Autodesk Inventor part; units mm, degrees
ref_plane "YZ Plane" through (0, 0, 0) normal (1, 0, 0) x (0, 1, 0)
ref_plane "XZ Plane" through (0, 0, 0) normal (0, 1, 0) x (-1, 0, 0)
ref_plane "XY Plane" through (0, 0, 0) normal (0, 0, 1) x (1, 0, 0)
sketch "Skizze1" plane through (0, 0, 0) normal (0, 0, 1) x (1, 0, 0)
  line L0 (0, 0) -> (0, 5.5)
  line L1 (0, 5.5) -> (5.6, 5.5)
  line L2 (5.6, 5.5) -> (5.6, 5)
  line L3 (5.6, 5) -> (13.6, 5)
  line L4 (13.6, 5) -> (13.6, 4.8)
  line L5 (13.6, 4.8) -> (14.7, 4.8)
  line L6 (14.7, 4.8) -> (14.7, 5)
  line L7 (14.7, 5) -> (15.3, 5)
  line L8 (15.8, 4.5) -> (15.8, 0)
  line L9 (15.8, 0) -> (0, 0)
  line L10 (0, 4) -> (-9.75, 4)
  line L11 (-11, 2.75) -> (-11, 0)
  line L12 (-11, 0) -> (0, 0)
  line L13 (15.3, 5) -> (15.8, 4.5)
  line L14 (-11, 2.75) -> (-9.75, 4)
  line L15 (1.5, 5.5) -> (1.5, 0) construction
  line L16 (13.6, 5) -> (13.6, 0) construction
  line L17 (4.6, 5.5) -> (4.6, 6)
  line L18 (4.6, 6) -> (0, 6)
  line L19 (0, 6) -> (0, 5.5)
  point P0 (15.8, 5)
  point P1 (-11, 4)
  dimension "d0" = 9.6
  dimension "d1" = 0.5
  dimension "d2" = 0.5
  dimension "d3" = 1.1
  dimension "d4" = 10
  dimension "d5" = 0.6
  dimension "d6" = 11
  dimension "d8" = 8
  dimension "d9" = 1.25
  dimension "d10" = 1.25
  dimension "d11" = 11
  dimension "d12" = 4.1
  dimension "d13" = 1.5
  dimension "d14" = 12.1
  dimension "d15" = 0
  dimension "d22" = 1
  dimension "d23" = 12
revolve "Umdrehung1" add sketch "Skizze1" angle 360 about axis through (15.8, 0, 0) along (-1, 0, 0) contours L12 L11 L14 L10 L0 | L0 L1 L2 L3 L4 L5 L6 L7 L13 L8 L9
thread "Gewinde1"
chamfer "Fase1" distance 0.1 angle 45 2 edges at (5.6, -5.5, 0) (0, -5.5, 0)
equation "\"d12\" = Bearing_StepThickness + SupportLink_Proximal_DistStep_Thickness"
equation "\"d14\" = Link_Thickness + SupportLink_Proximal_DistStep_Thickness"
equation "\"SupportLink_Proximal_DistStep_Thickness\" = 2.1"
properties part number "ParallelMech_SupportLink_Proximal_JointShaft"
Here's how the part is built. I have some questions about the finished solid (model axes, mm). A direction names the side the tool comes from. Round coordinates to 2 decimals unless told otherwise and drop trailing zeros. Order: outer loops, then holes, each group sorted by start corner. A loop starts at its lowest first (then second) coordinate and runs counter-clockwise, first axis right, second up. Notation, with made-up numbers: (-31.75, 7.5) -> (-17.75, 7.5) arc R26 cw to (-17.75, 24.5) -> close; hole circle Ø1 at (14, -35.75). An arc over 180 degrees is marked (long way). Use CSV: the item, a comma, the result in double quotes.
1. I need wall thicknesses on line 1 along Z through (x, y) = (-1.25, 0); line 2 along X through (y, z) = (2.5, -3.5); line 3 along X through (y, z) = (-4.75, 2.25). Which ranges of each line are inside material? Lowest first, please.
Recorded:
line 1,"z = -4 to 4"
line 2,"x = 0 to 15.8"
line 3,"x = 0 to 5.6"
2. I want a section at A-A on z = 0. List the corners of the cut face in (x, y) for me.
Recorded:
outline,"(-11, -2.75) -> (-9.75, -4) -> (0, -4) -> (0, -5.4) -> (0.1, -5.5) -> (5.5, -5.5) -> (5.6, -5.4) -> (5.6, -5) -> (13.6, -5) -> (13.6, -4.8) -> (14.7, -4.8) -> (14.7, -5) -> (15.3, -5) -> (15.8, -4.5) -> (15.8, 4.5) -> (15.3, 5) -> (14.7, 5) -> (14.7, 4.8) -> (13.6, 4.8) -> (13.6, 5) -> (5.6, 5) -> (5.6, 5.4) -> (5.5, 5.5) -> (0.1, 5.5) -> (0, 5.4) -> (0, 4) -> (-9.75, 4) -> (-11, 2.75) -> close"
3. I want a section at D-D on x = -0.75. List the corners of the cut face in (y, z) for me.
Recorded:
outline,"circle Ø8 at (0, 0)"
4. I want a section at C-C on x = 6.25. List the corners of the cut face in (y, z) for me.
Recorded:
outline,"circle Ø10 at (0, 0)"
5. I'm going to push flat-ended pins straight in: P1, Ø3, axis at x = -3.5, y = 1.5, coming from the -Z side; P2, Ø5, axis at x = -3, z = 2, coming from the +Y side; P3, Ø5, axis at x = 4.5, y = 1, coming from the +Z side; P4, Ø1.5, axis at x = -5.5, z = 4, coming from the -Y side. Where does each tip first touch, or does it pass through?
Recorded:
P1,"stops at z = -4"
P2,"stops at y = 4"
P3,"stops at z = 5.5"
P4,"stops at y = -2.33"
6. Thinking about a two-plate mould opening in X: for faces 1 (the face through (-11, 0, 0)), 2 (the face through (15, -1.08, -4.88)), 3 (the face through (14.16, 2.58, 4.05)), which applies, pulls with the +X half, pulls with the -X half, needs draft (parallel to the pull), parting line crosses it, or undercut?
Recorded:
face 1,"pulls with the -X half"
face 2,"needs draft"
face 3,"undercut"
7. Which directions (+Z, -Z, +X, -X, +Y, -Y) give clear straight access to the entire face, cutting with the end or side of a thin tool? Please do faces 4 (the face through (2.84, -1.19, -5.37)), 5 (the face through (0, -4, 2)), 6 (the face through (9.66, -1.08, -4.88)).
Recorded:
face 4,"+X, -X"
face 5,"-X"
face 6,"+X"
